The model under review builds one solid part; all positions refer to its coordinate system, in mm. A direction names the side the tool comes from. Round coordinates to 2 decimals unless told otherwise and drop trailing zeros. Write each loop counter-clockwise with the first axis right and the second up, starting at its lowest first coordinate (ties: lowest second). Pieces come first, ordered by that corner, then holes. Notation, with made-up numbers: (36.25, 40.5) - (73.25, 40.5) arc R18 cw to (73.25, 55.5) - close; hole circle Ø6 at (55.5, -7). An arc over 180 degrees is marked (long way). Return JSON: item names as keys, results as strings.
from build123d import *

# Parameters (mm, degrees)
EXTRUDE_4_DEPTH = 39
SKETCH_2_R      = 2.5
EXTRUDE_5_DEPTH = 8


with BuildPart() as part:
    # 草图1 → 凸台-拉伸4 (new body)
    with BuildSketch(Plane.XY):
        with BuildLine():
            ThreePointArc((11.999755772, 64.190702015), (7.19287537, 69.699227744), (0.441332655, 66.894477154))
            Line((0.441332655, 66.894477154), (-16.87917542, 36.894477154))
            Line((-16.87917542, 36.894477154), (-16.87917542, -3.105522846))
            Line((-16.87917542, -3.105522846), (-5.332170037, -23.105522846))
            Line((-5.332170037, -23.105522846), (9.992741519, -33.105522846))
            Line((9.992741519, -33.105522846), (11.999755772, -30.029791253))
            Line((11.999755772, -30.029791253), (-6.87917542, -3.105522846))
            Line((-6.87917542, -3.105522846), (-6.87917542, 14.190702015))
            Line((-6.87917542, 14.190702015), (-6.87917542, 24.190702015))
            Line((-6.87917542, 24.190702015), (10.114332844, 34.190702015))
            Line((10.114332844, 34.190702015), (11.999755772, 64.190702015))
        make_face()
    extrude(amount=EXTRUDE_4_DEPTH)

    # 草图2 → 凸台-拉伸5 (add)
    with BuildSketch(Plane.XY):
        with Locations((5.784422652, 63.881230161)):
            Circle(SKETCH_2_R)
    extrude(amount=-EXTRUDE_5_DEPTH)


solid = part.part
(1) Wall thickness on line 1 (Z direction, x = -4.5, y = 46); line 2 (X direction, y = 18, z = 17); line 3 (Y direction, x = -0.5, z = 33): over which ranges is each line inside the solid? List them lowest first.
Filled in:
{"line 1": "z = 0 to 39", "line 2": "x = -16.88 to -6.88", "line 3": "y = -26.26 to -12.2, 27.94 to 65.26"}
(2) Add section C-C (y = 20). Write out the cut boundary in (x, z).
Filled in:
{"outline": "(-16.88, 0) - (-6.88, 0) - (-6.88, 39) - (-16.88, 39) - close"}
(3) For faces 4 (the cylindrical face through (5.24, 61.44, -3.94)), 5 (the cylindrical face through (7.299, 69.673, 19.227)), 6 (the flat face through (2.692, -16.756, 19.227)), list the 3-axis set-ups (+Z, -Z, +X, -X, +Y, -Y) from which the entire face can be reached by the end or side of a thin tool; tool diameter is ignored.
Filled in:
{"face 4": "-Z", "face 5": "+Z, -Z, +Y", "face 6": "+Z, -Z, +X"}
(4) Add section B-B (z = 35). Write out the cut boundary in (x, y), plus the area to 3 significant figures.
Filled in:
{"outline": "(-16.88, -3.11) - (-5.33, -23.11) - (9.99, -33.11) - (12, -30.03) - (-6.88, -3.11) - (-6.88, 24.19) - (10.11, 34.19) - (12, 64.19) arc R6.26 ccw to (0.44, 66.89) - (-16.88, 36.89) - close", "area": "1,440 mm2"}
(5) Mouldability with a two-part tool opening along Y and no side actions: class faces 1 (the flat face through (-16.879, 17, 19)), 2 (the flat face through (2.223, -28.036, 19.227)), 3 (the flat face through (-6.879, 10, 19)) as released by +Y, released by -Y, zero draft, split by the parting line, or undercut.
Filled in:
{"face 1": "zero draft", "face 2": "released by -Y", "face 3": "undercut"}
(6) Clearance check with flat-ended pins moving along their axes: pin 1 Ø1.5 at (x, y) = (4, -19) entering from -Z; pin 2 Ø12 at (y, z) = (-17, 29) entering from -X; pin 3 Ø13.5 at (y, z) = (9, 20) entering from +X; pin 4 Ø8 at (x, y) = (1, 7.5) entering from -Z. State where each tip first meets the part, or that it passes through.
Filled in:
{"pin 1": "stops at z = 0", "pin 2": "stops at x = -12.32", "pin 3": "stops at x = -6.88", "pin 4": "passes through"}
(7) Add section A-A (x = -4). Write out the cut boundary in (y, z).
Filled in:
{"outline": "(-23.97, 0) - (-7.21, 0) - (-7.21, 39) - (-23.97, 39) - close; (25.88, 0) - (59.2, 0) - (59.2, 39) - (25.88, 39) - close"}
(8) Add section D-D (x = 5.25). Write out the cut boundary in (y, z).
Filled in:
{"outline": "(-30.01, 0) - (-20.4, 0) - (-20.4, 39) - (-30.01, 39) - close; (31.33, 0) - (61.44, 0) - (61.44, -8) - (66.32, -8) - (66.32, 0) - (69.84, 0) - (69.84, 39) - (31.33, 39) - close"}
